Check sheet for the modelled part. Datum: model origin and axes. Units: mm. Face numbers are marked on the shaded views. Round coordinates to 2 decimals unless told otherwise and drop trailing zeros. Order: outer loops, then holes, each group sorted by start corner. A loop starts at its lowest first (then second) coordinate and runs counter-clockwise, first axis right, second up.
```python
from build123d import *

# Parameters (mm, degrees)
SKETCH1_R            = 1.4
BOSS_EXTRUDE1_DEPTH  = 5
BOSS_EXTRUDE9_DEPTH  = 18.9
SKETCH1_4_R          = 1.4
CUT_EXTRUDE4_DEPTH   = 5
BOSS_EXTRUDE10_REACH = 49.608
SKETCH5_W            = 27.928634905
SKETCH5_H            = 3
SKETCH8_W            = 10
SKETCH8_H            = 21.9
SKETCH8_R            = 2
BOSS_EXTRUDE11_DEPTH = 3
SKETCH8_3_W          = 10
SKETCH8_3_H          = 21.9
BOSS_EXTRUDE12_DEPTH = 6
BOSS_EXTRUDE13_START = -3
BOSS_EXTRUDE13_DEPTH = 21.9
CUT_EXTRUDE5_DEPTH   = 6
BOSS_EXTRUDE14_DEPTH = 5
SKETCH11_2_W         = 8
SKETCH11_2_H         = 5
BOSS_EXTRUDE15_DEPTH = 3
SKETCH12_W           = 8
SKETCH12_H           = 5
CUT_EXTRUDE6_DEPTH   = 18.6


# Read off the part's stored shape, not the designer's step: Boss-Extrude9, Boss-Extrude13, Boss-Extrude14
with BuildPart() as part:
    # Sketch1 → Boss-Extrude1 (new body)
    with BuildSketch(Plane.XY):
        with BuildLine():
            Line((3.38, 2.541421507), (0, 2.523123532))
            Line((0, 2.523123532), (0, 0))
            Line((0, 0), (-29.5, 0))
            Line((-29.5, 0), (-29.5, 2.523123532))
            Line((-29.5, 2.523123532), (-32.88, 2.523123532))
            ThreePointArc((-32.88, 2.523123532), (-37.018209124, 6.273123532), (-32.88, 10.023123532))
            Line((-32.88, 10.023123532), (-29.5, 10.023123532))
            Line((-29.5, 10.023123532), (-29.5, 18.9))
            Line((-29.5, 18.9), (0, 18.9))
            Line((0, 18.9), (0, 10.023123532))
            Line((0, 10.023123532), (3.75, 10.023123532))
            ThreePointArc((3.75, 10.023123532), (7.495422713, 6.087897443), (3.38, 2.541421507))
        make_face()
        with Locations((3.75, 6.273123532)):
            Circle(SKETCH1_R, mode=Mode.SUBTRACT)
        with Locations((-33.25, 6.273123532)):
            Circle(SKETCH1_R, mode=Mode.SUBTRACT)
    extrude(amount=BOSS_EXTRUDE1_DEPTH)

    # Boss-Extrude9 outline → Boss-Extrude9 (add)
    with BuildSketch(Plane(origin=(0, 0, 0), x_dir=(1, 0, 0), z_dir=(0, 1, 0))):
        Polygon((0, -5), (12.051348998, -5), (8.550311307, 0), (0, 0), align=None)
    extrude(amount=BOSS_EXTRUDE9_DEPTH)

    # Sketch1<4> → Cut-Extrude4 (cut)
    with BuildSketch(Plane.XY):
        with Locations((3.75, 6.273123532)):
            Circle(SKETCH1_4_R)
    extrude(amount=CUT_EXTRUDE4_DEPTH, mode=Mode.SUBTRACT)

    # Boss-Extrude10: up to this face of the body (flat: up to its plane)
    boss_extrude10_end = Plane(part.part.faces().sort_by_distance((-10.115754309, 9.30291887, 5))[0])
    # Sketch5 → Boss-Extrude10 (add, up to the picked face)
    with BuildSketch(Plane(origin=(5.737345003, 0, -4.01733222), x_dir=(0.5735764363510504, 0, 0.8191520442889888), z_dir=(-0.8191520442889888, 0, 0.5735764363510504)), mode=Mode.PRIVATE) as boss_extrude10_sk1:
        with Locations((-2.95618742, -1.5)):
            Rectangle(SKETCH5_W, SKETCH5_H)
    boss_extrude10_tool1 = split(extrude(boss_extrude10_sk1.sketch, amount=BOSS_EXTRUDE10_REACH, mode=Mode.PRIVATE), bisect_by=boss_extrude10_end, keep=Keep.BOTH, mode=Mode.PRIVATE)
    add(boss_extrude10_tool1.solids().sort_by(Axis((4.041746, -1.5, -6.438899), (-0.8191520442889888, 0, 0.5735764363510504)))[0])



with BuildPart() as body_2:
    # Sketch8 → Boss-Extrude11 (new body)
    # profile 1 of 3: a face of its own
    with BuildSketch(Plane(origin=(5.737345003, 0, -4.01733222), x_dir=(0.5735764363510504, 0, 0.8191520442889888), z_dir=(-0.8191520442889888, 0, 0.5735764363510504))):
        with Locations((16.008130033, 7.95)):
            Rectangle(SKETCH8_W, SKETCH8_H)
        Polygon((19.408130033, 14.912990915), (16.008130033, 16.87598183), (12.608130033, 14.912990915), (12.608130033, 10.987009085), (16.008130033, 9.02401817), (19.408130033, 10.987009085), align=None, mode=Mode.SUBTRACT)
        Polygon((16.008130033, 6.87598183), (12.608130033, 4.912990915), (12.608130033, 0.987009085), (16.008130033, -0.97598183), (19.408130033, 0.987009085), (19.408130033, 4.912990915), align=None, mode=Mode.SUBTRACT)
    # profile 2 of 3: a face of its own
    with BuildSketch(Plane(origin=(5.737345003, 0, -4.01733222), x_dir=(0.5735764363510504, 0, 0.8191520442889888), z_dir=(-0.8191520442889888, 0, 0.5735764363510504))):
        Polygon((19.408130033, 4.912990915), (16.008130033, 6.87598183), (12.608130033, 4.912990915), (12.608130033, 0.987009085), (16.008130033, -0.97598183), (19.408130033, 0.987009085), align=None)
        with Locations(Location((16.008130033, 2.95, 0), (0, 0, 180))):
            Circle(SKETCH8_R, mode=Mode.SUBTRACT)
    # profile 3 of 3: a face of its own
    with BuildSketch(Plane(origin=(5.737345003, 0, -4.01733222), x_dir=(0.5735764363510504, 0, 0.8191520442889888), z_dir=(-0.8191520442889888, 0, 0.5735764363510504))):
        Polygon((19.408130033, 10.987009085), (19.408130033, 14.912990915), (16.008130033, 16.87598183), (12.608130033, 14.912990915), (12.608130033, 10.987009085), (16.008130033, 9.02401817), align=None)
        with Locations(Location((16.008130033, 12.95, 0), (0, 0, 180))):
            Circle(SKETCH8_R, mode=Mode.SUBTRACT)
    extrude(amount=BOSS_EXTRUDE11_DEPTH)

    # Sketch8<3> → Boss-Extrude12 (add)
    with BuildSketch(Plane(origin=(5.737345003, 0, -4.01733222), x_dir=(0.5735764363510504, 0, 0.8191520442889888), z_dir=(-0.8191520442889888, 0, 0.5735764363510504))):
        with Locations((16.008130033, 7.95)):
            Rectangle(SKETCH8_3_W, SKETCH8_3_H)
        Polygon((19.408130033, 14.912990915), (16.008130033, 16.87598183), (12.608130033, 14.912990915), (12.608130033, 10.987009085), (16.008130033, 9.02401817), (19.408130033, 10.987009085), align=None, mode=Mode.SUBTRACT)
        Polygon((16.008130033, 6.87598183), (12.608130033, 4.912990915), (12.608130033, 0.987009085), (16.008130033, -0.97598183), (19.408130033, 0.987009085), (19.408130033, 4.912990915), align=None, mode=Mode.SUBTRACT)
    extrude(amount=BOSS_EXTRUDE12_DEPTH)


with BuildPart() as part_1:
    add(part.part)

    add(body_2.part)  # Boss-Extrude13 merges body 2
    # Boss-Extrude13 outline → Boss-Extrude13 (add)
    with BuildSketch(Plane(origin=(0, 0, 0), x_dir=(1, 0, 0), z_dir=(0, 1, 0)).offset(BOSS_EXTRUDE13_START)):
        Polygon((12.051348998, -5), (4.726701466, -5), (7.136436733, -8.441458618), align=None)
    extrude(amount=BOSS_EXTRUDE13_DEPTH)

    # Sketch10 → Cut-Extrude5 (cut)
    with BuildSketch(Plane.XY.offset(5)):
        Polygon((2.104551733, 9.123123532), (0.459103466, 6.273123532), (2.104551733, 3.423123532), (5.395448267, 3.423123532), (7.040896534, 6.273123532), (5.395448267, 9.123123532), align=None)
    extrude(amount=CUT_EXTRUDE5_DEPTH, mode=Mode.SUBTRACT)

    # Boss-Extrude14 outline → Boss-Extrude14 (add)
    with BuildSketch(Plane.XY):
        with BuildLine():
            Line((-29.5, 10.023123532), (-29.5, 37.5))
            Line((-29.5, 37.5), (-37.5, 37.5))
            Line((-37.5, 37.5), (-37.5, 0))
            Line((-37.5, 0), (-29.5, 0))
            Line((-29.5, 0), (-29.5, 2.523123532))
            Line((-29.5, 2.523123532), (-32.88, 2.523123532))
            ThreePointArc((-32.88, 2.523123532), (-37.018209124, 6.273123532), (-32.88, 10.023123532))
            Line((-32.88, 10.023123532), (-29.5, 10.023123532))
        make_face()
    extrude(amount=BOSS_EXTRUDE14_DEPTH)

    # Sketch11<2> → Boss-Extrude15 (add)
    with BuildSketch(Plane(origin=(0, 0, 0), x_dir=(1, 0, 0), z_dir=(0, 1, 0))):
        with Locations((-33.5, -2.5)):
            Rectangle(SKETCH11_2_W, SKETCH11_2_H)
    extrude(amount=-BOSS_EXTRUDE15_DEPTH)

    # Sketch12 → Cut-Extrude6 (cut)
    with BuildSketch(Plane(origin=(0, 37.5, 0), x_dir=(1, 0, 0), z_dir=(0, 1, 0))):
        with Locations((-33.5, -2.5)):
            Rectangle(SKETCH12_W, SKETCH12_H)
    extrude(amount=-CUT_EXTRUDE6_DEPTH, mode=Mode.SUBTRACT)


solid = part_1.part
```
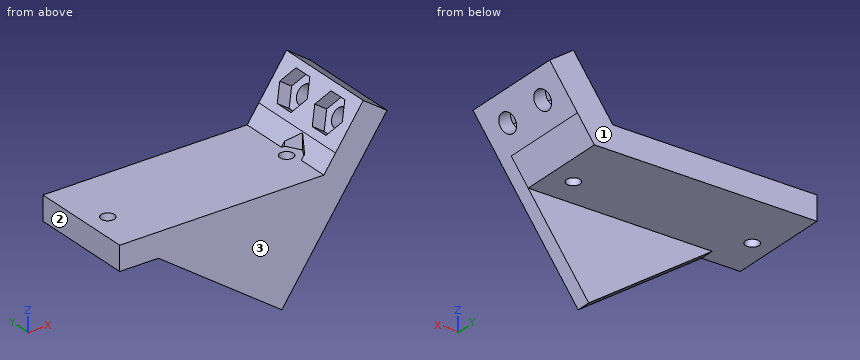
Item 1: Sectioned sample at A-A (x = -33.25). Record the cut outline in (y, z).
Answer:
outline: (-3, 0) - (4.87, 0) - (4.87, 5) - (-3, 5) - close; (7.67, 0) - (18.9, 0) - (18.9, 5) - (7.67, 5) - close
Item 2: Go/stop test with flat-tipped pins: P1, Ø1.5, axis at x = -3, y = 14, coming from the +Z side; P2, Ø6.5, axis at x = -15, y = 9, coming from the -Z side; P3, Ø8, axis at y = 15, z = -6.5, coming from the +X side; P4, Ø14.5, axis at x = -4, z = -11.5, coming from the +Y side. Record where each tip stops, or that it passes through.
Answer:
P1: stops at z = 5
P2: stops at z = 0
P3: passes through
P4: stops at y = 0
Item 3: Release check for a two-part mould opening along Y. For the marked faces 1, 2 and 3 record: released by +Y, released by -Y, zero draft, split by the parting line, or undercut.
Answer:
face 1: released by +Y
face 2: zero draft
face 3: released by -Y
Item 4: Sectioned sample at D-D (x = -9). Record the cut outline in (y, z), and give its area (3 significant figures).
Answer:
outline: (-3, -14.35) - (0, -14.35) - (0, 0) - (18.9, 0) - (18.9, 5) - (-3, 5) - close
area: 153 mm2
Item 5: Sectioned sample at C-C (x = 3.75). Record the cut outline in (y, z).
Answer:
outline: (-3, -6.86) - (0, -6.86) - (0, 0) - (4.87, 0) - (4.87, 5) - (-3, 5) - close; (7.67, 0) - (18.9, 0) - (18.9, 5) - (7.67, 5) - close
Item 6: Scan lines: line 1 along Y through (x, z) = (3.75, 3.2); line 2 along X through (y, z) = (6.5, 3); line 3 along X through (y, z) = (5, 2). Record each from-to range of solid material in increasing order.
Answer:
line 1: y = -3 to 4.87, 7.67 to 18.9
line 2: x = -37.5 to -34.63, -31.87 to 2.37, 5.13 to 10.65
line 3: x = -37.5 to -33.83, -32.67 to 3.17, 4.33 to 9.95
Item 7: Sectioned sample at B-B (y = 12). Record the cut outline in (x, z).
Answer:
outline: (-37.5, 0) - (8.55, 0) - (13.91, 7.65) - (11.45, 9.37) - (10.51, 8.03) - (8.05, 9.75) - (4.73, 5) - (-37.5, 5) - close; (11.95, 15.32) - (14.41, 13.6) - (13.47, 12.26) - (15.93, 10.54) - (17.79, 13.19) - (12.87, 16.63) - close
